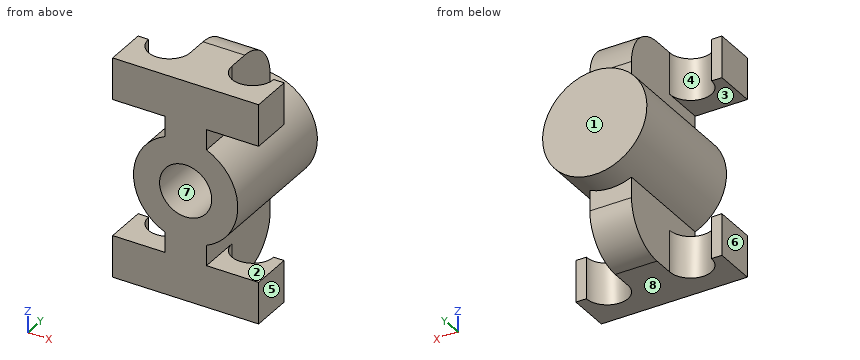
from build123d import *

# Parameters (mm, degrees)
SKETCH2_W                = 8
SKETCH2_H                = 42.16515139
BOSS_EXTRUDE3_DEPTH      = 20
BOSS_EXTRUDE4_DEPTH      = 5
BOSS_EXTRUDE4_DEPTH_BACK = 20
SKETCH4_R                = 10
HOLE1_D                  = 10
HOLE1_DEPTH              = 15
HOLE1_TIP                = 5
BOSS_EXTRUDE5_DEPTH      = 8
MIRROR3_COPY_1_DEPTH     = 8
FILLET1_R                = 8


with BuildPart() as part:
    # Sketch2 → Boss-Extrude3 (new body)
    with BuildSketch(Plane(origin=(0, 0, 0), x_dir=(1, 0, 0), z_dir=(0, 1, 0))):
        Rectangle(SKETCH2_W, SKETCH2_H)
    extrude(amount=BOSS_EXTRUDE3_DEPTH)

    # Sketch4 → Boss-Extrude4 (add, two sides: drawn at the far end of the back side and taken through both)
    with BuildSketch(Plane(origin=(0, 20, 0), x_dir=(-1, 0, 0), z_dir=(0, 1, 0)).offset(-BOSS_EXTRUDE4_DEPTH_BACK)):
        with Locations(Location((0, 0, 0), (0, 0, 90))):
            Circle(SKETCH4_R)
    extrude(amount=BOSS_EXTRUDE4_DEPTH + BOSS_EXTRUDE4_DEPTH_BACK)

    # Hole1
    with Locations(Plane.XZ):
        with Locations((0, 0)):
            Hole(HOLE1_D / 2, depth=HOLE1_DEPTH)
            with Locations((0, 0, -(HOLE1_DEPTH + HOLE1_TIP / 2))):  # 90° drill point
                Cone(0, HOLE1_D / 2, HOLE1_TIP, mode=Mode.SUBTRACT)

    # Sketch10 → Boss-Extrude5 (add)
    with BuildSketch(Plane.XY.offset(21.082575695)):
        with BuildLine():
            Line((-4, 0), (-14, 0))
            Line((-14, 0), (-14, 8))
            Line((-14, 8), (-12, 8))
            ThreePointArc((-12, 8), (-8, 4), (-4, 8))
            Line((-4, 8), (-4, 0))
        make_face()
    boss_extrude5 = extrude(amount=-BOSS_EXTRUDE5_DEPTH)

    # Mirror2: Boss-Extrude5 across plane
    add(boss_extrude5.mirror(Plane(origin=(0, 0, 0), x_dir=(0, 0, 1), z_dir=(1, 0, 0))))

    # Mirror3: Boss-Extrude5 across plane
    add(boss_extrude5.mirror(Plane.XY))

    # Mirror3 copy 1 sketch → Mirror3 copy 1 (add)
    with BuildSketch(Plane(origin=(0, 0, -21.082575695), x_dir=(-1, 0, 0), z_dir=(0, 0, -1))):
        with BuildLine():
            Line((-4, 0), (-14, 0))
            Line((-14, 0), (-14, 8))
            Line((-14, 8), (-12, 8))
            ThreePointArc((-12, 8), (-8, 4), (-4, 8))
            Line((-4, 8), (-4, 0))
        make_face()
    extrude(amount=-MIRROR3_COPY_1_DEPTH)

    # Fillet1
    fillet1_edges = [part.edges().sort_by_distance(p)[0] for p in [
        (0, 20, -21.082575695),
        (0, 20, 21.082575695),
    ]]
    fillet(fillet1_edges, radius=FILLET1_R)


solid = part.part
Work out the finished part from the listing and answer in its coordinate system (mm). Face numbers are marked on the shaded views. A direction names the side the tool comes from. Give positions to 0.01 mm unless a question says otherwise; leave off trailing zeros. Loops run counter-clockwise (first coordinate to the right, second up) from the corner with the lowest first, then second, coordinate; pieces in that order, holes last. Notation, with made-up numbers: (65, -12) -> (106, -12) arc R32 ccw to (106, 27) -> close; hole circle Ø3 at (60.5, 55). An arc over 180 degrees is marked (long way). Use a Markdown table: item, result. Add a question column.
1. Section B-B on x = 8 is taken. Determine the outline of the cut face in (y, z).
2. Flat-ended cylindrical pins translate along their axes: pin 1 Ø9 at (x, z) = (0, 0) entering from -Y; pin 2 Ø1.5 at (y, z) = (7, 10.5) entering from -X; pin 3 Ø1.6 at (x, z) = (-13.5, -16.5) entering from +Y. Find the tip coordinate at first contact, or state that the pin passes through.
3. Find the intervals of material crossed by probe 1 along X at (y, z) = (8, 0); probe 2 along Z at (x, y) = (8.5, 2.75); probe 3 along Z at (x, y) = (0, 7.5), in increasing order.
4. Section C-C on y = 10.5 is taken. Determine the outline of the cut face in (x, z), and give its area (3 significant figures).
5. Section D-D on z = -16 is taken. Determine the outline of the cut face in (x, y), and give its area (3 significant figures).
6. Section A-A on y = 6.5 is taken. State how many separate pieces and enclosed holes the cut face has, and give its area (3 significant figures).
7. Determine the mould class of the marked faces 6, 7 and 8 for opening direction Z: released by +Z, released by -Z, zero draft, split by the parting line, or undercut.
8. For the marked faces 1, 2, 3, 4 and 5, determine the directions among +Z, -Z, +X, -X, +Y, -Y from which every point of the face is accessible in a straight line to the end or side of a thin tool.
Results below:
| question | item | result |
|---|---|---|
| 1 | outline | (0, -21.08) -> (4, -21.08) -> (4, -13.08) -> (0, -13.08) -> close; (0, -6) -> (25, -6) -> (25, 6) -> (0, 6) -> close; (0, 13.08) -> (4, 13.08) -> (4, 21.08) -> (0, 21.08) -> close |
| 2 | pin 1 | stops at y = 15.5 |
| 2 | pin 2 | stops at x = -4 |
| 2 | pin 3 | stops at y = 8 |
| 3 | probe 1 | x = -10 to -5, 5 to 10 |
| 3 | probe 2 | z = -21.08 to -13.08, -5.27 to 5.27, 13.08 to 21.08 |
| 3 | probe 3 | z = -21.08 to -5, 5 to 21.08 |
| 4 | outline | (-4, -21.08) -> (4, -21.08) -> (4, -9.17) arc R10 ccw to (4, 9.17) -> (4, 21.08) -> (-4, 21.08) -> (-4, 9.17) arc R10 ccw to (-4, -9.17) -> close; hole circle Ø10 at (0, 0) |
| 4 | area | 417 mm^2 |
| 5 | outline | (-14, 0) -> (14, 0) -> (14, 8) -> (12, 8) arc R4 cw to (4, 8) -> (4, 19.45) -> (-4, 19.45) -> (-4, 8) arc R4 cw to (-12, 8) -> (-14, 8) -> close |
| 5 | area | 265 mm^2 |
| 6 | separate pieces | 5 |
| 6 | enclosed holes | 1 |
| 6 | area | 500 mm^2 |
| 7 | face 6 | zero draft |
| 7 | face 7 | undercut |
| 7 | face 8 | released by -Z |
| 8 | face 1 | +Z, -Z, +X, -X, +Y |
| 8 | face 2 | +X, +Y, -Y |
| 8 | face 3 | -X, +Y, -Y |
| 8 | face 4 | +Z, +Y |
| 8 | face 5 | +Z, -Z, +X, +Y, -Y |
